```python
from build123d import *

# Parameters (mm, degrees)
F1_DEPTH      = 3.5
F1_DEPTH_BACK = 3.5
F2_DEPTH      = 1.5
F2_DEPTH_BACK = 1.5
F3_R          = 1.99999
F4_T4_DEPTH   = 106.7758240051
F4_S5_R       = 15
F4_T6_DEPTH   = 55
F5_R          = 1.49999
F7_T1_DEPTH   = 11.00001
F7_T3_DEPTH   = 25.2313991783
F7_T5_DEPTH   = 21.00001
F7_T7_DEPTH   = 2e-05
F7_T10_ANGLE  = 90
F7_T12_ANGLE  = 90
F8_COUNT      = 2


# Not quite as in the source:
# - a fillet or chamfer that OpenCascade refuses, or shapes differently, is made with other operations: its cross-section is extruded or revolved along the edge and cut away or added
# - a fillet or chamfer is up to 0.001 mm smaller than in the source, because OpenCascade refuses the exact size
# - a feature names something its author has since deleted; it is built from what else it names


with BuildPart() as f1:
    # F0 (on Top) → F1 (new body, two sides)
    with BuildSketch(Plane.XY) as f1_sk:
        with BuildLine():
            ThreePointArc((-10, -5.0438080852), (-11.2, 0), (-10, 5.0438080852))
            Line((-10, 5.0438080852), (-10, 11.1803398875))
            ThreePointArc((-10, 11.1803398875), (-15, 0), (-10, -11.1803398875))
            Line((-10, -11.1803398875), (-10, -5.0438080852))
        make_face()
        with BuildLine():
            ThreePointArc((-10, 5.0438080852), (0, 11.2), (10, 5.0438080852))
            Line((10, 5.0438080852), (10, 11.1803398875))
            ThreePointArc((10, 11.1803398875), (0, 15), (-10, 11.1803398875))
            Line((-10, 11.1803398875), (-10, 5.0438080852))
        make_face()
        with BuildLine():
            ThreePointArc((10, 5.0438080852), (10.8958707775, 2.5922962794), (11.2, 0))
            ThreePointArc((11.2, 0), (10.8958707775, -2.5922962794), (10, -5.0438080852))
            Line((10, -5.0438080852), (10, -11.1803398875))
            ThreePointArc((10, -11.1803398875), (13.6930639376, -6.123724357), (15, 0))
            ThreePointArc((15, 0), (13.6930639376, 6.123724357), (10, 11.1803398875))
            Line((10, 11.1803398875), (10, 5.0438080852))
        make_face()
        with BuildLine():
            Line((10, -11.1803398875), (10, -5.0438080852))
            ThreePointArc((10, -5.0438080852), (0, -11.2), (-10, -5.0438080852))
            Line((-10, -5.0438080852), (-10, -11.1803398875))
            ThreePointArc((-10, -11.1803398875), (0, -15), (10, -11.1803398875))
        make_face()
    extrude(amount=F1_DEPTH)
    extrude(f1_sk.sketch, amount=-F1_DEPTH_BACK)

    # F0 (on Top) → F2 (join, two sides)
    with BuildSketch(Plane.XY) as f2_sk:
        with BuildLine():
            ThreePointArc((-10, 11.1803398875), (0, 15), (10, 11.1803398875))
            Line((10, 11.1803398875), (10, 40))
            Line((10, 40), (-10, 40))
            Line((-10, 40), (-10, 11.1803398875))
        make_face()
    extrude(amount=F2_DEPTH)
    extrude(f2_sk.sketch, amount=-F2_DEPTH_BACK)

    # F3 (radius 2 in the source; OpenCascade refuses exactly that, so slightly less here)
    f3_edges = [f1.edges().sort_by_distance(p)[0] for p in [
        (10, 11.18034, 3.5),
        (10, 11.18034, -3.5),
    ]]
    fillet(f3_edges, radius=F3_R)

    # F4: chamfer of 15 x 2.6449047106 on 1 edges, made by hand


with BuildPart() as f4_tool2:
    # F4_s3 → F4_t4 (new body)
    with BuildSketch(Plane.XZ.offset(27.7977420588)):
        Polygon((10, 1.1449047106), (-5, -1.5), (10, -1.5), align=None)
    extrude(amount=-F4_T4_DEPTH)

    # F4_s5 → F4_t6 (cut, symmetric)
    with BuildSketch(Plane.XY.offset(-0.2)):
        Circle(F4_S5_R)
    extrude(amount=F4_T6_DEPTH, both=True, mode=Mode.SUBTRACT)


with BuildPart() as f1_1:
    add(f1.part)

    # F4_t1: cut F4_tool2
    add(f4_tool2.part, mode=Mode.SUBTRACT)

    # F5 (radius 1.5 in the source; OpenCascade refuses exactly that, so slightly less here)
    f5_edges = [f1_1.edges().sort_by_distance(p)[0] for p in [
        (-10, 25.59017, -1.5),
        (-10, 25.59017, 1.5),
    ]]
    fillet(f5_edges, radius=F5_R)

    # F7: fillet of radius 1 on 6 edges, made by hand

    # F7_s2 → F7_t1 (cut)
    with BuildSketch(Plane.YZ.offset(-8.50001)):
        with BuildLine():
            ThreePointArc((40, -0.5), (39.7071067812, -1.2071067812), (39, -1.5))
            Line((39, -1.5), (40, -1.5))
            Line((40, -1.5), (40, -0.5))
        make_face()
    extrude(amount=F7_T1_DEPTH, mode=Mode.SUBTRACT)

    # F7_s4 → F7_t3 (cut)
    with BuildSketch(Plane(origin=(12.3562727231, 0, 2.178744262), x_dir=(0, 1, 0), z_dir=(-0.984807753, 0, -0.1736481777))):
        with BuildLine():
            ThreePointArc((40, -0.3910292588), (39.7071067812, 0.3160775224), (39, 0.6089707412))
            Line((39, 0.6089707412), (40, 0.6089707412))
            Line((40, 0.6089707412), (40, -0.3910292588))
        make_face()
    extrude(amount=F7_T3_DEPTH, mode=Mode.SUBTRACT)

    # F7_s6 → F7_t5 (cut)
    with BuildSketch(Plane.YZ.offset(-8.50001)):
        with BuildLine():
            ThreePointArc((39, 1.5), (39.7071067812, 1.2071067812), (40, 0.5))
            Line((40, 0.5), (40, 1.5))
            Line((40, 1.5), (39, 1.5))
        make_face()
    extrude(amount=F7_T5_DEPTH, mode=Mode.SUBTRACT)

    # F7_s8 → F7_t7 (cut)
    with BuildSketch(Plane.XY.offset(-1e-05)):
        with BuildLine():
            ThreePointArc((-10, 39), (-9.7071067812, 39.7071067812), (-9, 40))
            Line((-9, 40), (-10, 40))
            Line((-10, 40), (-10, 39))
        make_face()
    extrude(amount=F7_T7_DEPTH, mode=Mode.SUBTRACT)

    # F7_s9 → F7_t10 (revolve, cut)
    with BuildSketch(Plane.XY.offset(-1e-05)):
        with BuildLine():
            ThreePointArc((-9, 40), (-9.7071067812, 39.7071067812), (-10, 39))
            Line((-10, 39), (-10, 40))
            Line((-10, 40), (-9, 40))
        make_face()
    revolve(axis=Axis((-8.50001, 40, -1e-05), (0, -1, 0)), revolution_arc=F7_T10_ANGLE, mode=Mode.SUBTRACT)

    # F7_s11 → F7_t12 (revolve, cut)
    with BuildSketch(Plane.YZ.offset(-8.50001)):
        with BuildLine():
            ThreePointArc((39, 1.5), (39.7071067812, 1.2071067812), (40, 0.5))
            Line((40, 0.5), (40, 1.5))
            Line((40, 1.5), (39, 1.5))
        make_face()
    revolve(axis=Axis((-8.50001, 40, 1e-05), (0, -1, 0)), revolution_arc=F7_T12_ANGLE, mode=Mode.SUBTRACT)

    # F8: F1 ×2 about axis
    f8_axis = Axis((0, 0, -0.2721771598), (0, 0, -1))


with BuildPart() as f1_2:
    add(f1_1.part)
    for i in range(1, F8_COUNT):
        add(f1_1.part.rotate(f8_axis, i * 360 / F8_COUNT))


solid = f1_2.part
```
Read the model definition and answer for the solid it produces. Units are mm, in the model's axes. A direction names the side the tool comes from. Round coordinates to 2 decimals unless told otherwise and drop trailing zeros. Write each loop counter-clockwise with the first axis right and the second up, starting at its lowest first coordinate (ties: lowest second). Pieces come first, ordered by that corner, then holes. Notation, with made-up numbers: M -17,25 L 28,25 A21 cw 28,46 Z; hole C 79.5,-34 d10. An arc over 180 degrees is marked long. One line per item, written item: value.
Q1. Find section B-B on z = -2.25. Write down the section's boundary in (x, y), plus the area to 3 significant figures.
Data:
outline: C 0,0 d29.71; hole C 0,0 d22.4
area: 299 mm2
Q2. Which of the six approach directions +Z, -Z, +X, -X, +Y, -Y give full straight-line access (tool end or side, diameter ignored) to faces 1 (the cylindrical face through (-9.55, 24.9, 1.07)), 2 (the cylindrical face through (9.55, -24.9, 1.07)), 3 (the cylindrical face through (-9.57, 24.9, -1.05)), 4 (the cylindrical face through (-0.92, -39.58, -0.27)), 5 (the cylindrical face through (9.57, -24.9, -1.05))?
Data:
face 1: +Z, -X, +Y
face 2: +Z, +X, -Y
face 3: -Z, -X, +Y
face 4: -Z, -X, -Y
face 5: -Z, +X, -Y
Q3. Flat-ended cylindrical pins translate along their axes: pin 1 Ø3 at (x, y) = (6.5, -26) entering from -Z; pin 2 Ø9.5 at (x, y) = (-3.5, 23) entering from +Z; pin 3 Ø1 at (y, z) = (18.5, 0.5) entering from -X. Find the tip coordinate at first contact, or state that the pin passes through.
Data:
pin 1: z = -1.5
pin 2: z = 1.5
pin 3: x = -10
Q4. Straight lines are drawn through the part: line 1 (Z direction, x = -7.5, y = 29.5); line 2 (X direction, y = 3.5, z = 2.5); line 3 (Y direction, x = -6.5, z = -1.25). For each, find the intervals that lie inside material, in ascending order. Write a range as [from, to].
Data:
line 1: [-1.5, 1.5]
line 2: [-14.31, -10.64], [10.64, 14.31]
line 3: [-13.52, -9.12], [9.12, 39.66]
